Geometry: final body of the model. Coordinates: model frame, mm. A direction names the side the tool comes from. Coordinates: 2 decimals unless noted, no trailing zeros. Loops run counter-clockwise (first coordinate to the right, second up) from the corner with the lowest first, then second, coordinate; pieces in that order, holes last. Notation, with made-up numbers: M -14.75,59 L 1.25,59 A21 ccw 1.25,82 Z; hole C -5.5,65.5 d8. An arc over 180 degrees is marked long. Write item = value, one per line. Start each with the question number.
```python
from build123d import *

# Parameters (mm, degrees)
F1_DEPTH     = 15.24
F2_R         = 5.08
F3_R         = 5.08
F4_R         = 5.08
F5_S3_W      = 5.08
F5_S3_H      = 5.08
F5_T4_DEPTH  = 5.08
F5_T10_DEPTH = 102.9839018281


# Not quite as in the source:
# - a fillet or chamfer that OpenCascade refuses, or shapes differently, is made with other operations: its cross-section is extruded or revolved along the edge and cut away or added


with BuildPart() as f1:
    # F0 (on Top) → F1 (new body)
    with BuildSketch(Plane.XY):
        Polygon((-45.1973650922, 20.5321404808), (-35.0638359103, 20.5321404808), (-24.9303067284, 20.5321404808), (-27.7331978752, 25.3868903553), (-42.3944739453, 25.3868903553), align=None)
        Polygon((-24.9303067284, 20.5321404808), (-35.0638359103, 20.5321404808), (-35.0638359103, 20.5181515061), (-30.5441655604, 20.5181515061), (-26.0244952105, 12.6898528267), (-30.5441655604, 4.8615541473), (-35.0638359103, 4.8615541473), (-35.0638359103, 4.8475651727), (-24.9303067284, 4.8475651727), (-20.4025598402, 12.6898528267), align=None)
        Polygon((-27.7331978752, -0.0071847018), (-24.9303067284, 4.8475651727), (-35.0638359103, 4.8475651727), (-45.1973650922, 4.8475651727), (-42.3944739453, -0.0071847018), align=None)
        Polygon((70.4335950998, 20.5321404808), (-24.9303067284, 20.5321404808), (-20.4025598402, 12.6898528267), (-24.9303067284, 4.8475651727), (70.4335950998, 4.8475651727), align=None)
    extrude(amount=F1_DEPTH)

    # F2
    f2_edges = [f1.edges().sort_by_distance(p)[0] for p in [
        (70.433595, 20.53214, 7.62),
        (70.433595, 12.689853, 15.24),
    ]]
    fillet(f2_edges, radius=F2_R)

    # F3
    f3_edges = [f1.edges().sort_by_distance(p)[0] for p in [
        (70.433595, 10.149853, 0),
    ]]
    fillet(f3_edges, radius=F3_R)

    # F4
    f4_edges = [f1.edges().sort_by_distance(p)[0] for p in [
        (70.433595, 4.847565, 7.62),
    ]]
    fillet(f4_edges, radius=F4_R)

    # F5: fillet of radius 5.08 on 1 edges, made by hand


with BuildPart() as f5_tool2:
    # F5_s3 → F5_t4 (new body)
    with BuildSketch(Plane.XY.offset(10.16)):
        with Locations((67.8935950998, 17.9921404808)):
            Rectangle(F5_S3_W, F5_S3_H)
    extrude(amount=F5_T4_DEPTH)

    # F5_s5 → F5_t6 (revolve, cut)
    with BuildSketch(Plane(origin=(65.3535950998, 15.4521404808, 10.16), x_dir=(-0.7071067812, -0.7071067812, 0), z_dir=(-0.7071067812, 0.7071067812, 0))):
        with BuildLine():
            ThreePointArc((0, -5.08), (5.08, 0), (0, 5.08))
            Line((0, 5.08), (0, -5.08))
        make_face()
    revolve(axis=Axis((65.3535950998, 15.4521404808, 10.16), (0, 0, 1)), mode=Mode.SUBTRACT)


with BuildPart() as f1_1:
    add(f1.part)

    # F5_t1: cut F5_tool2
    add(f5_tool2.part, mode=Mode.SUBTRACT)


with BuildPart() as f5_tool8:
    # F5_s9 → F5_t10 (new body)
    with BuildSketch(Plane.YZ.offset(65.3535950998)):
        with BuildLine():
            ThreePointArc((15.4521404808, 15.24), (19.0442429292, 13.7521024484), (20.5321404808, 10.16))
            Line((20.5321404808, 10.16), (20.5321404808, 15.24))
            Line((20.5321404808, 15.24), (15.4521404808, 15.24))
        make_face()
    extrude(amount=-F5_T10_DEPTH)

    split(bisect_by=Plane(origin=(-9.8070524211, -5.6621043553, 0), x_dir=(0, 0, 1), z_dir=(0.8660254038, 0.5, 0)), keep=Keep.TOP)


with BuildPart() as f1_2:
    add(f1_1.part)

    # F5_t7: cut F5_tool8
    add(f5_tool8.part, mode=Mode.SUBTRACT)


solid = f1_2.part
```
Item 1: Section query C-C (x = 15). Return the cut outline in (y, z).
Item 2: Section query A-A (x = -37.5). Return the cut outline in (y, z), plus the area to 3 significant figures.
Item 3: First-contact query: pin 1 (10 mm diameter, centred on x = 13, y = 9, fed in from -Z); pin 2 (5.5 mm diameter, centred on x = 38.5, z = 7.5, fed in from -Y); pin 3 (2.5 mm diameter, centred on x = 30.5, z = 8, fed in from +Y); pin 4 (3 mm diameter, centred on y = 12, z = 10.5, fed in from -X). Flat tips, straight axial feed; report the tip coordinate or a pass-through.
Item 4: Line query: line 1 (Y direction, x = -33, z = 3); line 2 (Y direction, x = 59, z = 5); line 3 (Y direction, x = -28, z = 1.75). Output: solid intervals per line, ascending. Write a range as from..to.
Item 5: Reachability of faces 1 (the cylindrical face through (20.844, 19.005, 13.791)), 2 (the cylindrical face through (19.58, 6.296, 13.712)), 3 (the flat face through (-33, 20.518, 8)), 4 (the cylindrical face through (20.844, 6.296, 1.528)), 5 (the flat face through (20, 4.848, 8)) from +Z, -Z, +X, -X, +Y, -Y: full face, straight path, thin tool, end or side. Return the list, or none.
Item 6: Section query D-D (y = 18.75). Return the cut outline in (x, z).
Verdict:
q1.outline = M 4.85,5.08 A5.08 ccw 9.93,0 L 15.45,0 A5.08 ccw 20.53,5.08 L 20.53,10.16 A5.08 ccw 15.45,15.24 L 9.93,15.24 A5.08 ccw 4.85,10.16 Z
q2.outline = M -0.01,0 L 4.85,0 L 4.85,15.24 L -0.01,15.24 Z; M 20.53,0 L 25.39,0 L 25.39,15.24 L 20.53,15.24 Z
q2.area = 148 mm2
q3.pin_1 = 0
q3.pin_2 = 4.85
q3.pin_3 = 20.53
q3.pin_4 = -27.29
q4.line_1 = -0.01..4.86, 20.52..25.39
q4.line_2 = 4.85..20.53
q4.line_3 = -0.01..9.27, 16.11..25.39
q5.face_1 = +Z, +X, +Y
q5.face_2 = +Z, +X, -Y
q5.face_3 = +Z, -Z, -X
q5.face_4 = -Z, +X, -Y
q5.face_5 = +Z, -Z, +X, -Y
q6.outline = M -29.52,0 L -23.9,0 L -23.9,1.22 L 65.35,1.22 A3.86 ccw 69.22,5.08 L 69.22,10.16 A3.86 ccw 65.35,14.02 L -23.9,14.02 L -23.9,15.24 L -29.52,15.24 Z
